Design review of the part built by this model. Coordinates are the model's own, in mm. A direction names the side the tool comes from. Coordinates: 2 decimals unless noted, no trailing zeros. Loops run counter-clockwise (first coordinate to the right, second up) from the corner with the lowest first, then second, coordinate; pieces in that order, holes last. Notation, with made-up numbers: (6, -29.75) -> (22, -29.75) arc R33 ccw to (22, 4.25) -> close; hole circle Ø2 at (14, 89). An arc over 180 degrees is marked (long way). Answer in a Markdown table with one row per item.
```python
from build123d import *

# Parameters (mm, degrees)
SKETCH2_R           = 5
BOSS_EXTRUDE1_DEPTH = 3
SKETCH3_R           = 1
CUT_EXTRUDE1_DEPTH  = 10
SKETCH5_R           = 1
CUT_EXTRUDE2_DEPTH  = 10
CUT_EXTRUDE3_START  = -10
SKETCH6_R           = 1
CUT_EXTRUDE3_DEPTH  = 10


with BuildPart() as part:
    # Sketch2 → Boss-Extrude1 (new body)
    with BuildSketch(Plane.XY):
        with BuildLine():
            Line((117, 140), (117, 120))
            Line((117, 120), (237, 120))
            Line((237, 120), (237, 0))
            Line((237, 0), (0, 0))
            Line((0, 0), (0, 170))
            Line((0, 170), (87, 170))
            ThreePointArc((87, 170), (108.213203436, 161.213203436), (117, 140))
        make_face()
        with Locations((50, 11.25)):
            Circle(SKETCH2_R, mode=Mode.SUBTRACT)
        with Locations((177, 11.25)):
            Circle(SKETCH2_R, mode=Mode.SUBTRACT)
        with BuildLine():
            Line((30, 155), (87, 155))
            ThreePointArc((87, 155), (94, 148), (87, 141))
            Line((87, 141), (30, 141))
            ThreePointArc((30, 141), (23, 148), (30, 155))
        make_face(mode=Mode.SUBTRACT)
    extrude(amount=BOSS_EXTRUDE1_DEPTH)

    # Sketch3 → Cut-Extrude1 (cut)
    with BuildSketch(Plane.ZY):
        with Locations((1.5, 168.5)):
            Circle(SKETCH3_R)
        with Locations((1.5, 1.5)):
            Circle(SKETCH3_R)
    extrude(amount=-CUT_EXTRUDE1_DEPTH, mode=Mode.SUBTRACT)

    # Sketch5 → Cut-Extrude2 (cut)
    with BuildSketch(Plane.ZY):
        with Locations((1.5, 50)):
            Circle(SKETCH5_R)
    extrude(amount=-CUT_EXTRUDE2_DEPTH, mode=Mode.SUBTRACT)

    # Sketch6 → Cut-Extrude3 (cut)
    with BuildSketch(Plane(origin=(237, 0, 0), x_dir=(0, 0, -1), z_dir=(1, 0, 0)).offset(CUT_EXTRUDE3_START)):
        with Locations((-1.5, 118.5)):
            Circle(SKETCH6_R)
        with Locations(Location((-1.5, 1.5, 0), (0, 0, 180))):
            Circle(SKETCH6_R)
        with Locations(Location((-1.5, 50, 0), (0, 0, 180))):
            Circle(SKETCH6_R)
    extrude(amount=CUT_EXTRUDE3_DEPTH, mode=Mode.SUBTRACT)


solid = part.part
```
(1) To check wall thickness, follow probe 1 along Y at (x, z) = (69.5, 1.85); probe 2 along Y at (x, z) = (177, 0.7); probe 3 along Z at (x, y) = (232, 118). State the ranges of each line that lie inside material, in increasing order.
Evaluation:
| item | result |
|---|---|
| probe 1 | y = 0 to 141, 155 to 170 |
| probe 2 | y = 0 to 6.25, 16.25 to 120 |
| probe 3 | z = 0 to 0.63, 2.37 to 3 |
(2) Take a section at A-A on x = 50. Give the boundary of the cut face in (y, z), and give its area (3 significant figures).
Evaluation:
| item | result |
|---|---|
| outline | (0, 0) -> (6.25, 0) -> (6.25, 3) -> (0, 3) -> close; (16.25, 0) -> (141, 0) -> (141, 3) -> (16.25, 3) -> close; (155, 0) -> (170, 0) -> (170, 3) -> (155, 3) -> close |
| area | 438 mm² |
(3) Take a section at B-B on y = 11.25. Give the boundary of the cut face in (x, z), and give its area (3 significant figures).
Evaluation:
| item | result |
|---|---|
| outline | (0, 0) -> (45, 0) -> (45, 3) -> (0, 3) -> close; (55, 0) -> (172, 0) -> (172, 3) -> (55, 3) -> close; (182, 0) -> (237, 0) -> (237, 3) -> (182, 3) -> close |
| area | 651 mm² |
(4) For pin 1 (1.5 mm diameter, centred on y = 126, z = 1, fed in from +X); pin 2 (1 mm diameter, centred on y = 1.5, z = 1.5, fed in from -X); pin 3 (0.6 mm diameter, centred on y = 118.5, z = 1.5, fed in from +X), all flat-tipped, find the tip position at first contact; note any pin that passes through.
Evaluation:
| item | result |
|---|---|
| pin 1 | stops at x = 117 |
| pin 2 | stops at x = 10 |
| pin 3 | stops at x = 227 |
(5) Take a section at C-C on z = 1.25. Count the separate pieces of the cut face and the enclosed holes in it, and give its area (3 significant figures).
Evaluation:
| item | result |
|---|---|
| separate pieces | 1 |
| enclosed holes | 3 |
| area | 32,900 mm² |
(6) Draft analysis for pull direction Y (two halves, no side actions). For faces 1 (the cylindrical face through (107.979, 161.445, 1.479)), 2 (the cylindrical face through (94, 148, 1)), 3 (the flat face through (120, 67, 3)), state which applies: pulls with the +Y half, pulls with the -Y half, needs draft (parallel to the pull), parting line crosses it, or undercut.
Evaluation:
| item | result |
|---|---|
| face 1 | pulls with the +Y half |
| face 2 | undercut |
| face 3 | needs draft |
(7) Tool access review of faces 4 (the flat face through (120, 67, 0)), 5 (the cylindrical face through (23, 148, 1)): name each direction out of +Z, -Z, +X, -X, +Y, -Y from which nothing blocks a thin tool from reaching the whole face with its end or side.
Evaluation:
| item | result |
|---|---|
| face 4 | -Z, +X, -X, +Y, -Y |
| face 5 | +Z, -Z |
(8) Take a section at D-D on y = 125. Give the boundary of the cut face in (x, z), and give its area (3 significant figures).
Evaluation:
| item | result |
|---|---|
| outline | (0, 0) -> (117, 0) -> (117, 3) -> (0, 3) -> close |
| area | 351 mm² |
